The figure shows three views and two pictorial views of one solid part (mm, origin at its lowest corner). Answer the questions. A direction names the side the tool comes from. Coordinates: 2 decimals unless noted, no trailing zeros. Order: outer loops, then holes, each group sorted by start corner. A loop starts at its lowest first (then second) coordinate and runs counter-clockwise, first axis right, second up. Notation, with made-up numbers: M 84,44.5 L 110,44.5 A21 cw 110,73.5 Z; hole C -9.75,63 d1. An arc over 180 degrees is marked long. Use a Markdown table: item, result.
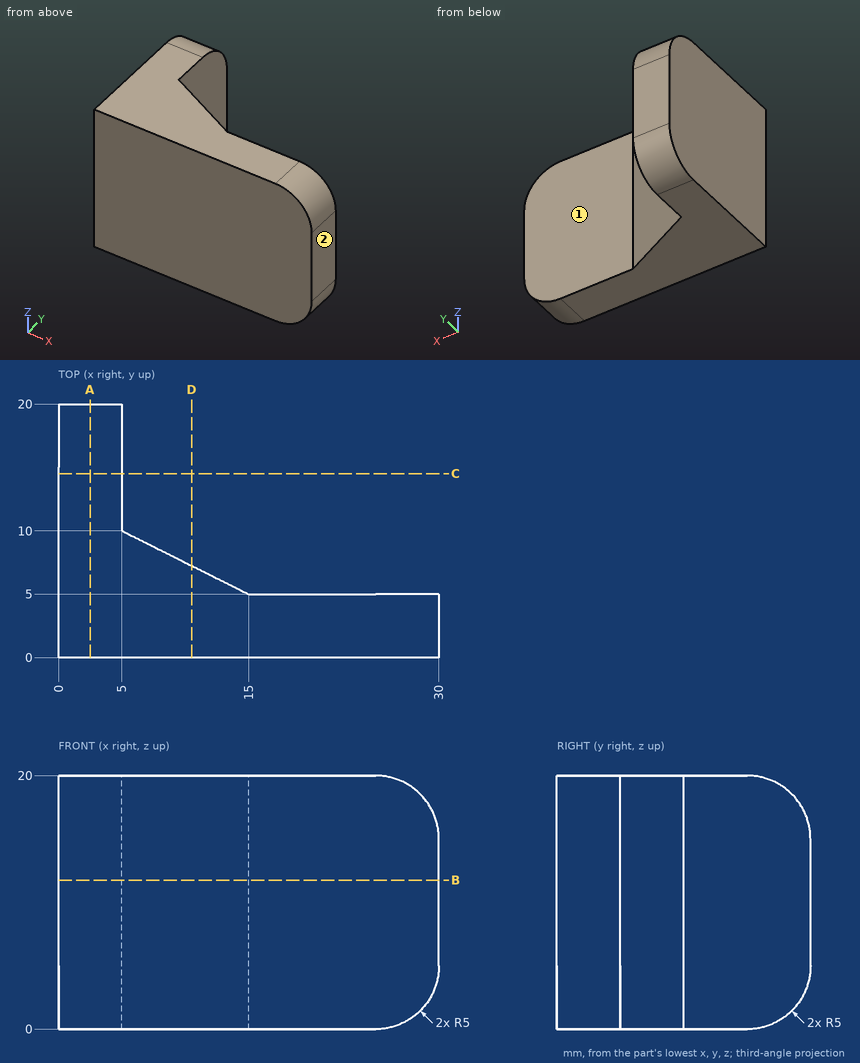
1. For the marked faces 1 and 2, determine the directions among +Z, -Z, +X, -X, +Y, -Y from which every point of the face is accessible in a straight line to the end or side of a thin tool.
Answers below:
| item | result |
|---|---|
| face 1 | +Z, -Z, +X, +Y |
| face 2 | +Z, -Z, +X, +Y, -Y |
2. Find the intervals of material crossed by probe 1 along Y at (x, z) = (26.75, 9.75); probe 2 along X at (y, z) = (9.5, 7), in increasing order.
Answers below:
| item | result |
|---|---|
| probe 1 | 0 to 5 |
| probe 2 | 0 to 6 |
3. Section C-C on y = 14.5 is taken. Determine the outline of the cut face in (x, z).
Answers below:
| item | result |
|---|---|
| outline | M 0,0 L 5,0 L 5,20 L 0,20 Z |
4. Section A-A on x = 2.5 is taken. Determine the outline of the cut face in (y, z), then the cut area to 3 significant figures.
Answers below:
| item | result |
|---|---|
| outline | M 0,0 L 15,0 A5 ccw 20,5 L 20,15 A5 ccw 15,20 L 0,20 Z |
| area | 389 mm² |
5. Flat-ended cylindrical pins translate along their axes: P1, Ø8, axis at y = 14, z = 3, coming from the -X side; P2, Ø6, axis at x = 16, z = 4, coming from the +Y side; P3, Ø12, axis at x = 23.5, y = 15, coming from the +Z side; P4, Ø8, axis at y = 18, z = 9, coming from the +X side. Find the tip coordinate at first contact, or state that the pin passes through.
Answers below:
| item | result |
|---|---|
| P1 | x = 0 |
| P2 | y = 6 |
| P3 | through |
| P4 | x = 5 |
6. Section B-B on z = 11.75 is taken. Determine the outline of the cut face in (x, y).
Answers below:
| item | result |
|---|---|
| outline | M 0,0 L 30,0 L 30,5 L 15,5 L 5,10 L 5,20 L 0,20 Z |
7. Section D-D on x = 10.5 is taken. Determine the outline of the cut face in (y, z).
Answers below:
| item | result |
|---|---|
| outline | M 0,0 L 7.25,0 L 7.25,20 L 0,20 Z |
